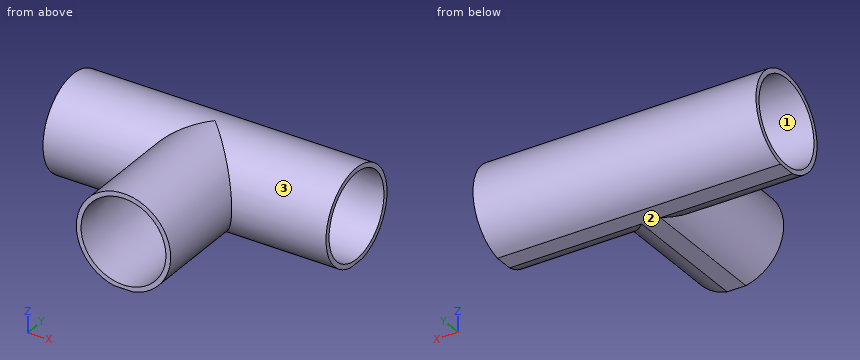
from build123d import *

# Parameters (mm, degrees)
F4_COUNT      = 3
F4_ANGLE      = 180
F5_W          = 152.4
F5_H          = 0.508
F6_DEPTH      = 76.2010001
F6_DEPTH_BACK = 76.2010001


with BuildPart() as f1:
    # F0 (on Front) → F1 (revolve)
    with BuildSketch(Plane.XZ):
        Polygon((76.2, 25.4), (0, 25.4), (0, 21.717), (76.2, 22.86), align=None)
    revolve(axis=Axis((-51.9470935156, 0, 0), (-1, 0, 0)))

    # F4: F1 ×3 about axis
    f4_axis = Axis((0, 0, 5.3851941696), (0, 0, -1))


with BuildPart() as f1_1:
    add(f1.part)
    for i in range(1, F4_COUNT):
        add(f1.part.rotate(f4_axis, i * F4_ANGLE / (F4_COUNT - 1)))

    # F5 (on Right) → F6 (cut, two sides)
    with BuildSketch(Plane.YZ) as f6_sk:
        with Locations((-50.8, -25.146)):
            Rectangle(F5_W, F5_H)
    extrude(amount=-F6_DEPTH, mode=Mode.SUBTRACT)
    extrude(f6_sk.sketch, amount=F6_DEPTH_BACK, mode=Mode.SUBTRACT)


solid = f1_1.part
Build history of the part. All positions in model axes, mm. Face numbers are marked on the shaded views. Coordinates: 2 decimals unless noted, no trailing zeros. Order: outer loops, then holes, each group sorted by start corner. A loop starts at its lowest first (then second) coordinate and runs counter-clockwise, first axis right, second up. Notation, with made-up numbers: (55, 37.25) -> (88, 37.25) arc R25 cw to (88, 64.25) -> close; hole circle Ø4 at (1, 26). An arc over 180 degrees is marked (long way). One line per item, written item: value.
(1) Slice it at A-A, the plane y = -69.5. List the corners of the cut face in (x, z).
Checked values:
outline: (-5.05, -24.89) -> (5.05, -24.89) arc R25.4 ccw (long way) to start; hole circle Ø45.52 at (0, 0)
(2) Drop flat-ended pins along their axis: pin 1 Ø12 at (x, z) = (-56.5, 8) entering from +Y; pin 2 Ø20.5 at (x, z) = (-10, -10.5) entering from +Y; pin 3 Ø1.5 at (x, y) = (4, -61) entering from +Z; pin 4 Ø12 at (y, z) = (-26, -5.5) entering from +X. Give the stop position or say it passes through.
Checked values:
pin 1: y = 25.32
pin 2: y = 25.4
pin 3: z = 25.19
pin 4: x = 76.2
(3) Slice it at B-B, the plane x = -29.5. List the corners of the cut face in (y, z), plus the area to 3 significant figures.
Checked values:
outline: (-5.05, -24.89) -> (5.05, -24.89) arc R25.4 ccw (long way) to start; hole circle Ø44.32 at (0, 0)
area: 481 mm2
(4) Mould opens along Y. For the marked faces 1, 2 and 3 say: pulls with the +Y half, pulls with the -Y half, needs draft (parallel to the pull), parting line crosses it, or undercut.
Checked values:
face 1: undercut
face 2: needs draft
face 3: parting line crosses it
(5) Probe line 1 (Z direction, x = -51.5, y = 13); line 2 (Y direction, x = 43, z = -17); line 3 (Z direction, x = 66.5, y = -8). List the from-to ranges inside material, lowest first. Write a range as [from, to].
Checked values:
line 1: [-21.82, -18.35], [18.35, 21.82]
line 2: [-18.87, -14.53], [14.53, 18.87]
line 3: [-24.11, -21.26], [21.26, 24.11]
